```python
from build123d import *

# Parameters (mm, degrees)
F0_R     = 16.51
F1_DEPTH = 6.35
F2_R     = 12.6746
F3_DEPTH = 2.54
F4_R     = 10.6426
F5_DEPTH = 3.556
F6_R     = 12.6746
F7_DEPTH = 2.54
F8_R     = 0.127
F9_SIZE  = 0.508


with BuildPart() as f1:
    # F0 (on Top) → F1 (new body)
    with BuildSketch(Plane.XY):
        Circle(F0_R)
    extrude(amount=F1_DEPTH)

    # F2 (on face) → F3 (join)
    with BuildSketch(Plane.XY.offset(6.35)):
        Circle(F2_R)
    extrude(amount=F3_DEPTH)

    # F4 (on face) → F5 (join)
    with BuildSketch(Plane.XY.offset(8.89)):
        Circle(F4_R)
    extrude(amount=F5_DEPTH)

    # F6 (on face) → F7 (join)
    with BuildSketch(Plane.XY.offset(12.446)):
        Circle(F6_R)
    extrude(amount=F7_DEPTH)

    # F8
    f8_edges = [f1.edges().sort_by_distance(p)[0] for p in [
        (-10.6426, 0, 8.89),
        (-12.6746, 0, 8.89),
        (-12.6746, 0, 12.446),
        (-10.6426, 0, 12.446),
    ]]
    fillet(f8_edges, radius=F8_R)

    # F9
    f9_edges = [f1.edges().sort_by_distance(p)[0] for p in [
        (-12.6746, 0, 14.986),
    ]]
    chamfer(f9_edges, length=F9_SIZE)


solid = f1.part
```
Geometry: final body of the model. Coordinates: model frame, mm. A direction names the side the tool comes from. Round coordinates to 2 decimals unless told otherwise and drop trailing zeros. Order: outer loops, then holes, each group sorted by start corner. A loop starts at its lowest first (then second) coordinate and runs counter-clockwise, first axis right, second up. Notation, with made-up numbers: M 65.5,-7 L 80.5,-7 A14 cw 80.5,18 Z; hole C 83,7 d2. An arc over 180 degrees is marked long. Use one line per item in the form item = value. Start each with the question number.
Q1. Pin query (flat end, axial travel): pin 1 Ø1.5 at (y, z) = (10.5, 4) entering from -X; pin 2 Ø3 at (x, z) = (6.5, 3) entering from -Y; pin 3 Ø2 at (x, z) = (6.5, 3.5) entering from -Y. Return the tip coordinate at first contact, or that it passes through.
Q2. Mould query, pull axis X, two halves, no side actions, for faces 1 (the face through (-10.06, -7.71, 7.54)), 2 (the face through (3.7, 10.3, 12.446)). Classes: +X half, -X half, draft (parallel to the pull), parting line (faces both ways), or undercut.
Q3. Material intervals for line 1 (Z direction, x = 5, y = 15.5); line 2 (Y direction, x = 0.5, z = 12.75); line 3 (Y direction, x = 0, z = 12.25), sorted ascending. Write a range as [from, to].
Q4. Access query for faces 3 (the face through (-10.06, -7.71, 13.51)), 4 (the face through (15.748, 4.959, 3.131)), 5 (the face through (-2.31, -10.39, 10.64)). Directions: +Z, -Z, +X, -X, +Y, -Y. A direction counts if a zero-diameter tool reaches every point of the face in a straight line with its end or side. Return the directions, or none.
Q5. Cut plane C-C (z = 2). Return loops of the section in (x, y).
Q6. Cut plane D-D (z = 10). Return loops of the section in (x, y), and give its area (3 significant figures).
Q7. Cut plane A-A (y = 0). Return loops of the section in (x, z).
Geometry results:
q1.pin_1 = -13.32
q1.pin_2 = -15.73
q1.pin_3 = -15.57
q2.face_1 = parting line
q2.face_2 = draft
q3.line_1 = [0, 6.35]
q3.line_2 = [-12.66, 12.66]
q3.line_3 = [-10.64, 10.64]
q4.face_3 = +Z
q4.face_4 = +Z, -Z
q4.face_5 = none
q5.outline = C 0,0 d33.02
q6.outline = C 0,0 d21.29
q6.area = 356 mm^2
q7.outline = M -16.51,0 L 16.51,0 L 16.51,6.35 L 12.67,6.35 L 12.67,8.76 A0.13 ccw 12.55,8.89 L 10.77,8.89 A0.13 cw 10.64,9.02 L 10.64,12.32 A0.13 cw 10.77,12.45 L 12.55,12.45 A0.13 ccw 12.67,12.57 L 12.67,14.48 L 12.17,14.99 L -12.17,14.99 L -12.67,14.48 L -12.67,12.57 A0.13 ccw -12.55,12.45 L -10.77,12.45 A0.13 cw -10.64,12.32 L -10.64,9.02 A0.13 cw -10.77,8.89 L -12.55,8.89 A0.13 ccw -12.67,8.76 L -12.67,6.35 L -16.51,6.35 Z
